from build123d import *

# Parameters (mm, degrees)
SKETCH1_R           = 63.5
BOSS_EXTRUDE1_DEPTH = 5.08
BOSS_EXTRUDE2_DEPTH = 12.7
SKETCH5_R           = 3.175
CUT_EXTRUDE1_DEPTH  = 6.08
SKETCH6_R           = 3.302
CUT_EXTRUDE2_DEPTH  = 18.78


with BuildPart() as part:
    # Sketch1 → Boss-Extrude1 (new body)
    with BuildSketch(Plane(origin=(0, 0, 0), x_dir=(1, 0, 0), z_dir=(0, 1, 0))):
        Circle(SKETCH1_R)
    extrude(amount=BOSS_EXTRUDE1_DEPTH)

    # Sketch2 → Boss-Extrude2 (add)
    with BuildSketch(Plane(origin=(0, 5.08, 0), x_dir=(1, 0, 0), z_dir=(0, 1, 0))):
        with BuildLine():
            Line((-5.113329796, 8.779490782), (0, 0))
            Line((0, 0), (10.159926948, 0.03852811))
            ThreePointArc((10.159926948, 0.03852811), (-5.046597152, -8.818018893), (-5.113329796, 8.779490782))
        make_face()
    extrude(amount=BOSS_EXTRUDE2_DEPTH)

    # Sketch5 → Cut-Extrude1 (cut, through all)
    with BuildSketch(Plane(origin=(0, 5.08, 0), x_dir=(1, 0, 0), z_dir=(0, 1, 0))):
        with Locations((2.628439651, 5.021053822)):
            Circle(SKETCH5_R)
    extrude(amount=-CUT_EXTRUDE1_DEPTH, mode=Mode.SUBTRACT)

    # Sketch6 → Cut-Extrude2 (cut, through all)
    with BuildSketch(Plane(origin=(0, 17.78, 0), x_dir=(1, 0, 0), z_dir=(0, 1, 0))):
        with Locations((-2.432656569, -4.122340405)):
            Circle(SKETCH6_R)
    extrude(amount=-CUT_EXTRUDE2_DEPTH, mode=Mode.SUBTRACT)


solid = part.part
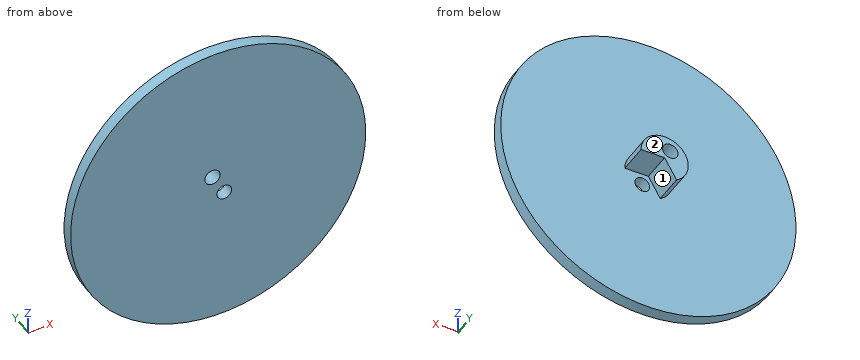
Work out the finished part from the listing and answer in its coordinate system (mm). Face numbers are marked on the shaded views. A direction names the side the tool comes from. Coordinates: 2 decimals unless noted, no trailing zeros. Write each loop counter-clockwise with the first axis right and the second up, starting at its lowest first coordinate (ties: lowest second). Pieces come first, ordered by that corner, then holes.
1. Consider line 1 along Y through (x, z) = (-39.5, -48.5); line 2 along Z through (x, y) = (-5, 1.75); line 3 along X through (y, z) = (8.25, 2.5). Determine where each line is inside the solid, lowest interval first.
Results list:
line 1: y = 0 to 5.08
line 2: z = -63.3 to 2.05, 6.2 to 63.3
line 3: x = -9.85 to -5.31, 0.44 to 9.85
2. The part is cut by section D-D, the plane y = 2.25. Write down the section's boundary in (x, z) (3 decimals), and give its area (3 significant figures).
Results list:
outline: circle Ø127 at (0, 0); hole circle Ø6.604 at (-2.433, 4.122); hole circle Ø6.35 at (2.628, -5.021)
area: 12,600 mm2
3. The part is cut by section C-C, the plane z = -35. Write down the section's boundary in (x, y).
Results list:
outline: (-52.98, 0) - (52.98, 0) - (52.98, 5.08) - (-52.98, 5.08) - close
4. For the marked faces 1 and 2, determine the directions among +Z, -Z, +X, -X, +Y, -Y from which every point of the face is accessible in a straight line to the end or side of a thin tool.
Results list:
face 1: -Z, +X, +Y
face 2: +Z, -Z, +X, -X, +Y
5. The part is cut by section B-B, the plane x = 36.5. Write down the section's boundary in (y, z).
Results list:
outline: (0, -51.96) - (5.08, -51.96) - (5.08, 51.96) - (0, 51.96) - close
6. Flat-ended cylindrical pins translate along their axes: pin 1 (1 mm diameter, centred on y = 5, z = -30.5, fed in from +X); pin 2 (6 mm diameter, centred on x = 32, y = 4, fed in from -Z); pin 3 (3 mm diameter, centred on y = 6.5, z = 3.5, fed in from +X). Find the tip coordinate at first contact, or state that the pin passes through.
Results list:
pin 1: stops at x = 55.97
pin 2: stops at z = -56.49
pin 3: stops at x = 63.43
7. The part is cut by section A-A, the plane y = 12.75. Write down the section's boundary in (x, z).
Results list:
outline: (-5.11, -8.78) - (0, 0) - (10.16, -0.04) arc R10.16 ccw (long way) to start; hole circle Ø6.6 at (-2.43, 4.12)
